Check sheet for the modelled part. Datum: model origin and axes. Units: mm. A direction names the side the tool comes from. Coordinates: 2 decimals unless noted, no trailing zeros. Use CSV: the item, a comma, the result in double quotes. Start each with the question number.
1. Thickness scan on L1, parallel to X at y = -1, z = 1; L2, parallel to Z at x = -18.5, y = -37; L3, parallel to X at y = 0, z = 8. Record the ranges inside material, lowest first.
2. Gauge pin test, flat ends, axial feed: pin 1 (5 mm diameter, centred on y = -7, z = 6, fed in from -X); pin 2 (2 mm diameter, centred on x = -33.5, z = 7, fed in from -Y); pin 3 (2 mm diameter, centred on x = -33.5, y = 17.5, fed in from -Z). Record the tip position at first contact, or that the pin passes through.
3. Set-up check for faces 1 (the face through (-1, 9, 10)), 2 (the face through (-28, 21, 3)): record each of +Z, -Z, +X, -X, +Y, -Y from which the full face is reachable in a straight line by a thin tool's end or side.
```python
from build123d import *

# Parameters (mm, degrees)
F2_R = 1


with BuildPart() as f1:
    # F0 (on Front) → F1 (revolve)
    with BuildSketch(Plane.XZ):
        with BuildLine():
            Line((0, 5), (0, 0))
            Line((0, 0), (35, 0))
            Line((35, 0), (35, 5))
            Line((35, 5), (45, 5))
            Line((45, 5), (45, 10))
            Line((45, 10), (5, 10))
            ThreePointArc((5, 10), (3.535534, 6.464466), (0, 5))
        make_face()
    revolve(axis=Axis((0, 0, 5), (0, 0, -1)))

    # F2
    f2_edges = [f1.edges().sort_by_distance(p)[0] for p in [
        (-45, 0, 10),
    ]]
    fillet(f2_edges, radius=F2_R)


solid = f1.part
```
Completed:
1,L1,"-34.99 to 34.99"
1,L2,"5 to 10"
1,L3,"-45 to -4.58, 4.58 to 45"
2,pin 1,"x = -44.77"
2,pin 2,"y = -31.12"
2,pin 3,"z = 5"
3,face 1,"+Z, +X, -X, +Y, -Y"
3,face 2,"-Z"
